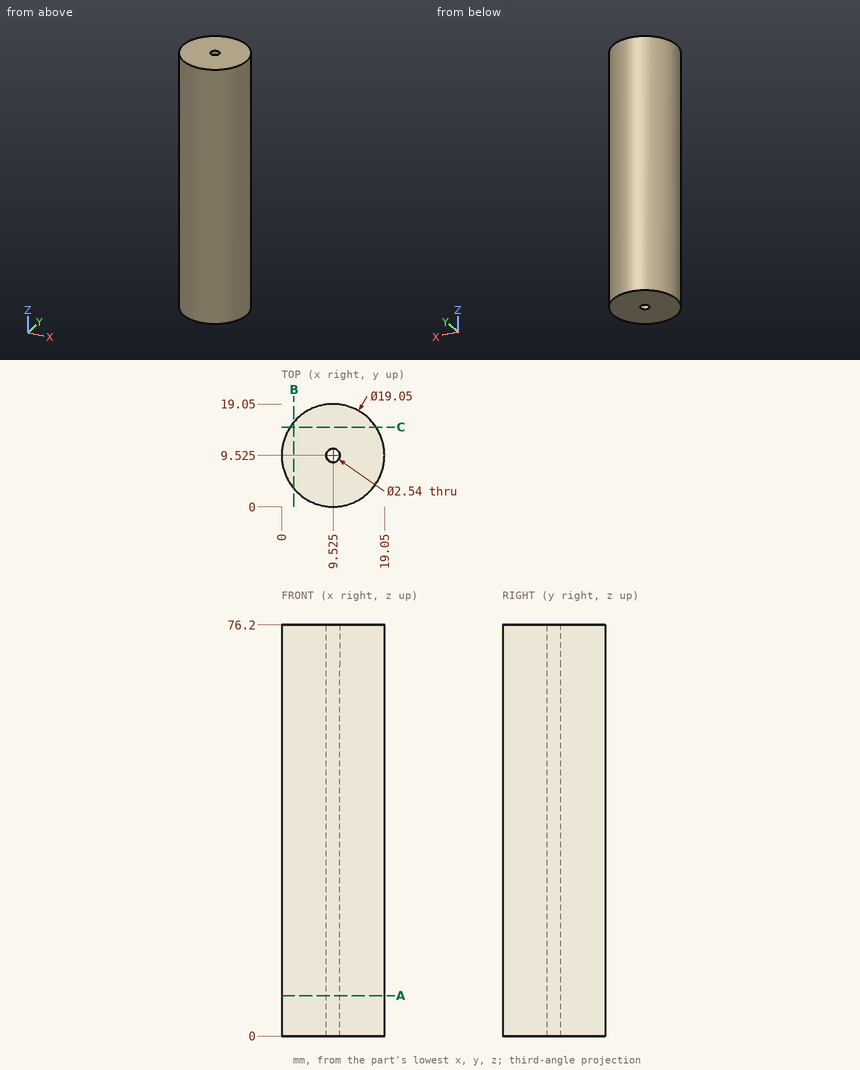
Could you check a few things on this drawing? It's one solid part, dimensions in mm from its lowest x, y, z. Coordinates: 2 decimals unless noted, no trailing zeros. Write each loop counter-clockwise with the first axis right and the second up, starting at its lowest first coordinate (ties: lowest second). Pieces come first, ordered by that corner, then holes. Notation, with made-up numbers: (-29, 86.25) - (9, 86.25) arc R31 cw to (9, 124.25) - close; hole circle Ø4 at (78.25, -31.75). An arc over 180 degrees is marked (long way). Put each result on its own line as item: value. Start each with the question number.
Q1. Please list where these lines run through material, in increasing order: L1, parallel to Y at x = 8.5, z = 71; L2, parallel to Y at x = 10, z = 7; L3, parallel to X at y = 9, z = 53.
Q2. I want a section at A-A on z = 7.5. Write out the boundary of the cut face in (x, y) (3 decimals).
Q3. I want a section at B-B on x = 2.25. Write out the boundary of the cut face in (y, z), plus the area to 3 significant figures.
Q4. I'm going to push flat-ended pins straight in: P1, Ø1, axis at x = 3, z = 57, coming from the +Y side; P2, Ø1.5, axis at x = 10.5, z = 66.5, coming from the -Y side; P3, Ø1.5, axis at x = 2.5, z = 12, coming from the -Y side. Where does each tip first touch, or does it pass through?
Q5. I want a section at C-C on y = 14.75. Write out the boundary of the cut face in (x, z).
Checks:
1. L1: 0.06 to 8.78, 10.27 to 18.99
1. L2: 0.01 to 8.35, 10.7 to 19.04
1. L3: 0.01 to 8.37, 10.68 to 19.04
2. outline: circle Ø19.05 at (9.525, 9.525); hole circle Ø2.54 at (9.525, 9.525)
3. outline: (3.38, 0) - (15.67, 0) - (15.67, 76.2) - (3.38, 76.2) - close
3. area: 937 mm²
4. P1: y = 16.9
4. P2: y = 0
4. P3: y = 2.36
5. outline: (1.56, 0) - (17.49, 0) - (17.49, 76.2) - (1.56, 76.2) - close
